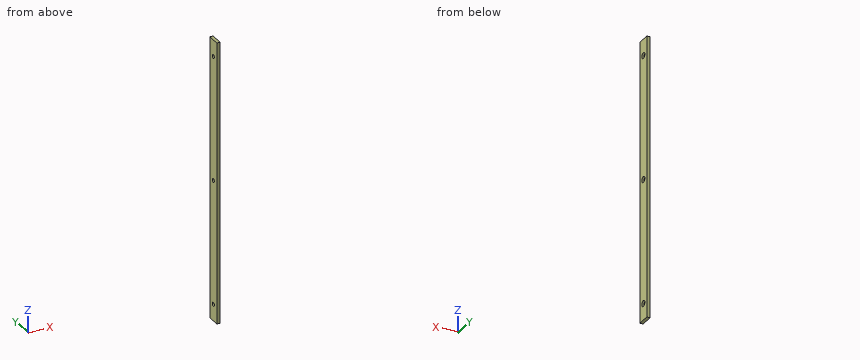
```python
from build123d import *

# Parameters (mm, degrees)
SKETCH_W        = 10
SKETCH_H        = 40
PAD_DEPTH       = 850
SKETCH001_R     = 6
POCKET_DEPTH    = 10.001
SKETCH002_R     = 9
POCKET001_DEPTH = 6


with BuildPart() as part:
    # Sketch → Pad (new body)
    with BuildSketch(Plane.XY):
        with Locations((5, 20)):
            Rectangle(SKETCH_W, SKETCH_H)
    extrude(amount=PAD_DEPTH)

    # Sketch001 (on Face4 of Pad) → Pocket (cut, through all)
    with BuildSketch(Plane(origin=(0, 0, 0), x_dir=(0, -1, 0), z_dir=(-1, 0, 0))):
        with Locations((-20, 50)):
            Circle(SKETCH001_R)
        with Locations((-20, 425)):
            Circle(SKETCH001_R)
        with Locations((-20, 800)):
            Circle(SKETCH001_R)
    extrude(amount=-POCKET_DEPTH, mode=Mode.SUBTRACT)

    # Sketch002 (on Face3 of Pocket) → Pocket001 (cut)
    with BuildSketch(Plane.YZ.offset(10)):
        with Locations((20, 800)):
            Circle(SKETCH002_R)
        with Locations((20, 425)):
            Circle(SKETCH002_R)
        with Locations((20, 50)):
            Circle(SKETCH002_R)
    extrude(amount=-POCKET001_DEPTH, mode=Mode.SUBTRACT)


solid = part.part
```
Source: CAD feature listing. Evaluate the final solid. Frame: model axes, mm. Round coordinates to 2 decimals unless told otherwise and drop trailing zeros. Order: outer loops, then holes, each group sorted by start corner. A loop starts at its lowest first (then second) coordinate and runs counter-clockwise, first axis right, second up. Notation, with made-up numbers: (50, 58.25) -> (76, 58.25) arc R17 ccw to (76, 89.25) -> close; hole circle Ø2 at (35, 42.5). An arc over 180 degrees is marked (long way). One line per item, written item: value. Start each with the question number.
Q1. Pin query (flat end, axial travel): pin 1 (14.5 mm diameter, centred on y = 23, z = 426.5, fed in from +X); pin 2 (16 mm diameter, centred on y = 20, z = 50, fed in from +X). Return the tip coordinate at first contact, or that it passes through.
Q2. Material intervals for probe 1 along Z at (x, y) = (1.65, 20); probe 2 along Y at (x, z) = (1.2, 425); probe 3 along Z at (x, y) = (8.25, 12), sorted ascending.
Q3. Section query A-A (y = 20). Return the cut outline in (x, z).
Findings below:
1. pin 1: x = 10
1. pin 2: x = 4
2. probe 1: 0 to 44, 56 to 419, 431 to 794, 806 to 850
2. probe 2: 0 to 14, 26 to 40
2. probe 3: 0 to 45.88, 54.12 to 420.88, 429.12 to 795.88, 804.12 to 850
3. outline: (0, 0) -> (10, 0) -> (10, 41) -> (4, 41) -> (4, 44) -> (0, 44) -> close; (0, 56) -> (4, 56) -> (4, 59) -> (10, 59) -> (10, 416) -> (4, 416) -> (4, 419) -> (0, 419) -> close; (0, 431) -> (4, 431) -> (4, 434) -> (10, 434) -> (10, 791) -> (4, 791) -> (4, 794) -> (0, 794) -> close; (0, 806) -> (4, 806) -> (4, 809) -> (10, 809) -> (10, 850) -> (0, 850) -> close
